```python
from build123d import *

# Parameters (mm, degrees)
SKETCH1_R          = 4.5
BASE_FLANGE1_DEPTH = 3
CHAMFER2_SIZE      = 15
CHAMFER3_SIZE      = 2


# Sheet-metal steps are written as plain solids
with BuildPart() as part:
    # Sketch1 → Base-Flange1 (new body)
    with BuildSketch(Plane.XY):
        Polygon((-5.322794555, 29.058388501), (23.677205445, 29.058388501), (36.677205445, 29.058388501), (36.677205445, -24.941611499), (17.443611724, -24.941611499), (-5.322794555, -24.941611499), (-5.322794555, -12.941611499), (-8.322794555, -12.941611499), (-8.322794555, -24.941611499), (-20.322794555, -24.941611499), (-20.322794555, 29.058388501), (-8.322794555, 29.058388501), (-8.322794555, 17.058388501), (-5.322794555, 17.058388501), align=None)
        with Locations((23.677205445, 2.058388501)):
            Circle(SKETCH1_R, mode=Mode.SUBTRACT)
    extrude(amount=-BASE_FLANGE1_DEPTH)

    # Chamfer2
    chamfer2_edges = [part.edges().sort_by_distance(p)[0] for p in [
        (36.677205445, 29.058388501, -1.5),
        (36.677205445, -24.941611499, -1.5),
    ]]
    chamfer(chamfer2_edges, length=CHAMFER2_SIZE)

    # Chamfer3
    chamfer3_edges = [part.edges().sort_by_distance(p)[0] for p in [
        (-8.322794555, -24.941611499, -1.5),
        (-8.322794555, 29.058388501, -1.5),
    ]]
    chamfer(chamfer3_edges, length=CHAMFER3_SIZE)


solid = part.part
```
Model file for the job. Use its own axes, mm. A direction names the side the tool comes from. Give positions to 0.01 mm unless a question says otherwise; leave off trailing zeros. Loops run counter-clockwise (first coordinate to the right, second up) from the corner with the lowest first, then second, coordinate; pieces in that order, holes last. Notation, with made-up numbers: (-7, -9.75) -> (31, -9.75) arc R17 cw to (31, -1.75) -> close; hole circle Ø2 at (58, -37.5). An arc over 180 degrees is marked (long way). Use CSV: the item, a comma, the result in double quotes. Start each with the question number.
1) Mould opens along Y. For faces 1 (the flat face through (-7, 17.058, -1)), 2 (the cylindrical face through (27.97, 3.41, -1.48)), 3 (the flat face through (8, -24.942, -1)) say: released by +Y, released by -Y, zero draft, split by the parting line, or undercut.
2) Slice it at A-A on y = -18. Give the cut face in (x, z), plus the area to 3 significant figures.
3) Wall check: line 1 (X direction, y = 6, z = -1.1); line 2 (X direction, y = 1, z = -0.25); line 3 (Y direction, x = 23, z = -0.85). Give the ranges that are in metal, low to high.
4) Tool access for faces 4 (the flat face through (-9.337, 28.072, -1.479)), 5 (the flat face through (-15, 29.058, -1)), 6 (the flat face through (-8.323, -18, -1)): list every direction of +Z, -Z, +X, -X, +Y, -Y with a clear straight run to the whole face (end or side of a thin tool).
5) Slice it at C-C on z = -2.1. Give the cut face in (x, y).
6) Slice it at D-D on y = 16. Give the cut face in (x, z).
7) Slice it at B-B on x = 25. Give the cut face in (y, z), plus the area to 3 significant figures.
8) Flat gauge pins, fed straight in: pin 1 Ø1.5 at (y, z) = (22, -1) entering from +X; pin 2 Ø1.5 at (x, z) = (-7.5, -2) entering from +Y; pin 3 Ø1.5 at (x, z) = (27, -2) entering from +Y. Where does each tip first touch, or does it go through?
Computed values:
1,face 1,"released by +Y"
1,face 2,"undercut"
1,face 3,"released by -Y"
2,outline,"(-20.32, -3) -> (-8.32, -3) -> (-8.32, 0) -> (-20.32, 0) -> close; (-5.32, -3) -> (28.62, -3) -> (28.62, 0) -> (-5.32, 0) -> close"
2,area,"138 mm^2"
3,line 1,"x = -20.32 to 21.51, 25.85 to 36.68"
3,line 2,"x = -20.32 to 19.3, 28.05 to 36.68"
3,line 3,"y = -23.62 to -2.39, 6.51 to 27.74"
4,face 4,"+Z, -Z, +Y"
4,face 5,"+Z, -Z, +X, -X, +Y"
4,face 6,"+Z, -Z, -Y"
5,outline,"(-20.32, -24.94) -> (-10.32, -24.94) -> (-8.32, -22.94) -> (-8.32, -12.94) -> (-5.32, -12.94) -> (-5.32, -24.94) -> (21.68, -24.94) -> (36.68, -9.94) -> (36.68, 14.06) -> (21.68, 29.06) -> (-5.32, 29.06) -> (-5.32, 17.06) -> (-8.32, 17.06) -> (-8.32, 27.06) -> (-10.32, 29.06) -> (-20.32, 29.06) -> close; hole circle Ø9 at (23.68, 2.06)"
6,outline,"(-20.32, -3) -> (34.74, -3) -> (34.74, 0) -> (-20.32, 0) -> close"
7,outline,"(-21.62, -3) -> (-2.24, -3) -> (-2.24, 0) -> (-21.62, 0) -> close; (6.36, -3) -> (25.74, -3) -> (25.74, 0) -> (6.36, 0) -> close"
7,area,"116 mm^2"
8,pin 1,"stops at x = 29.49"
8,pin 2,"stops at y = 17.06"
8,pin 3,"stops at y = 24.49"
